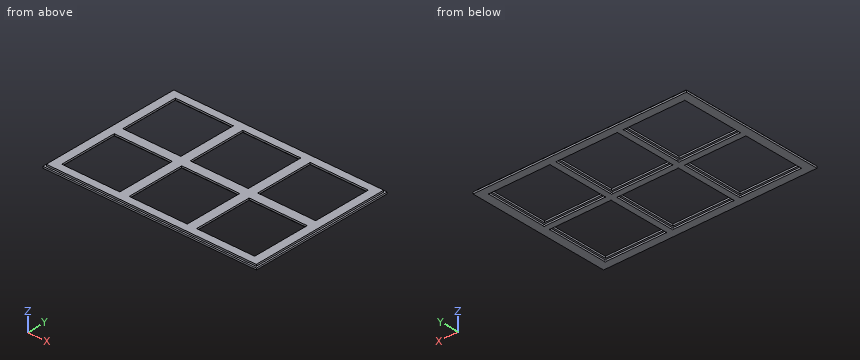
from build123d import *

# Parameters (mm, degrees)
SKETCH1_W           = 1250
SKETCH1_H           = 845
BOSS_EXTRUDE1_DEPTH = 20
SKETCH2_W           = 360
SKETCH2_H           = 360
CUT_EXTRUDE1_DEPTH  = 10
SKETCH3_W           = 340
SKETCH3_H           = 340
CUT_EXTRUDE2_DEPTH  = 11
SKETCH4_W           = 1250
SKETCH4_H           = 845
SKETCH4_W_2         = 1230
SKETCH4_H_2         = 825
CUT_EXTRUDE3_DEPTH  = 10


with BuildPart() as part:
    # Sketch1 → Boss-Extrude1 (new body)
    with BuildSketch(Plane.XY):
        Rectangle(SKETCH1_W, SKETCH1_H)
    extrude(amount=BOSS_EXTRUDE1_DEPTH)

    # Sketch2 → Cut-Extrude1 (cut)
    with BuildSketch(Plane(origin=(0, 0, 0), x_dir=(-1, 0, 0), z_dir=(0, 0, -1))):
        with Locations((-395, 197.5)):
            Rectangle(SKETCH2_W, SKETCH2_H)
        with BuildLine():
            Line((-575, 372.627718677), (-575, 377.5))
            Line((-575, 377.5), (-570.127718677, 377.5))
            ThreePointArc((-570.127718677, 377.5), (-575.474873734, 377.974873734), (-575, 372.627718677))
        make_face()
        with BuildLine():
            ThreePointArc((-215, 372.627718677), (-214.525126266, 377.974873734), (-219.872281323, 377.5))
            Line((-219.872281323, 377.5), (-215, 377.5))
            Line((-215, 377.5), (-215, 372.627718677))
        make_face()
        with BuildLine():
            Line((-180, 372.627718677), (-180, 377.5))
            Line((-180, 377.5), (-175.127718677, 377.5))
            ThreePointArc((-175.127718677, 377.5), (-180.474873734, 377.974873734), (-180, 372.627718677))
        make_face()
        with BuildLine():
            Line((-575, 17.5), (-575, 22.372281323))
            ThreePointArc((-575, 22.372281323), (-575.474873734, 17.025126266), (-570.127718677, 17.5))
            Line((-570.127718677, 17.5), (-575, 17.5))
        make_face()
        with BuildLine():
            ThreePointArc((-219.872281323, 17.5), (-214.525126266, 17.025126266), (-215, 22.372281323))
            Line((-215, 22.372281323), (-215, 17.5))
            Line((-215, 17.5), (-219.872281323, 17.5))
        make_face()
        with BuildLine():
            Line((-180, 17.5), (-180, 22.372281323))
            ThreePointArc((-180, 22.372281323), (-180.474873734, 17.025126266), (-175.127718677, 17.5))
            Line((-175.127718677, 17.5), (-180, 17.5))
        make_face()
        with Locations((0, 197.5)):
            Rectangle(SKETCH2_W, SKETCH2_H)
        with BuildLine():
            Line((180, 17.5), (175.127718677, 17.5))
            ThreePointArc((175.127718677, 17.5), (180.474873734, 17.025126266), (180, 22.372281323))
            Line((180, 22.372281323), (180, 17.5))
        make_face()
        with BuildLine():
            Line((175.127718677, -17.5), (180, -17.5))
            Line((180, -17.5), (180, -22.372281323))
            ThreePointArc((180, -22.372281323), (180.474873734, -17.025126266), (175.127718677, -17.5))
        make_face()
        with BuildLine():
            Line((215, -17.5), (219.872281323, -17.5))
            ThreePointArc((219.872281323, -17.5), (214.525126266, -17.025126266), (215, -22.372281323))
            Line((215, -22.372281323), (215, -17.5))
        make_face()
        with BuildLine():
            Line((215, 17.5), (215, 22.372281323))
            ThreePointArc((215, 22.372281323), (214.525126266, 17.025126266), (219.872281323, 17.5))
            Line((219.872281323, 17.5), (215, 17.5))
        make_face()
        with Locations((395, 197.5)):
            Rectangle(SKETCH2_W, SKETCH2_H)
        with BuildLine():
            ThreePointArc((180, 372.627718677), (180.474873734, 377.974873734), (175.127718677, 377.5))
            Line((175.127718677, 377.5), (180, 377.5))
            Line((180, 377.5), (180, 372.627718677))
        make_face()
        with BuildLine():
            Line((215, 372.627718677), (215, 377.5))
            Line((215, 377.5), (219.872281323, 377.5))
            ThreePointArc((219.872281323, 377.5), (214.525126266, 377.974873734), (215, 372.627718677))
        make_face()
        with BuildLine():
            ThreePointArc((575, 372.627718677), (575.474873734, 377.974873734), (570.127718677, 377.5))
            Line((570.127718677, 377.5), (575, 377.5))
            Line((575, 377.5), (575, 372.627718677))
        make_face()
        with BuildLine():
            Line((575, 17.5), (570.127718677, 17.5))
            ThreePointArc((570.127718677, 17.5), (575.474873734, 17.025126266), (575, 22.372281323))
            Line((575, 22.372281323), (575, 17.5))
        make_face()
        with BuildLine():
            Line((570.127718677, -17.5), (575, -17.5))
            Line((575, -17.5), (575, -22.372281323))
            ThreePointArc((575, -22.372281323), (575.474873734, -17.025126266), (570.127718677, -17.5))
        make_face()
        with Locations((395, -197.5)):
            Rectangle(SKETCH2_W, SKETCH2_H)
        with BuildLine():
            ThreePointArc((570.127718677, -377.5), (575.474873734, -377.974873734), (575, -372.627718677))
            Line((575, -372.627718677), (575, -377.5))
            Line((575, -377.5), (570.127718677, -377.5))
        make_face()
        with BuildLine():
            Line((215, -377.5), (215, -372.627718677))
            ThreePointArc((215, -372.627718677), (214.525126266, -377.974873734), (219.872281323, -377.5))
            Line((219.872281323, -377.5), (215, -377.5))
        make_face()
        with BuildLine():
            ThreePointArc((175.127718677, -377.5), (180.474873734, -377.974873734), (180, -372.627718677))
            Line((180, -372.627718677), (180, -377.5))
            Line((180, -377.5), (175.127718677, -377.5))
        make_face()
        with Locations((0, -197.5)):
            Rectangle(SKETCH2_W, SKETCH2_H)
        with BuildLine():
            Line((-180, -17.5), (-175.127718677, -17.5))
            ThreePointArc((-175.127718677, -17.5), (-180.474873734, -17.025126266), (-180, -22.372281323))
            Line((-180, -22.372281323), (-180, -17.5))
        make_face()
        with BuildLine():
            Line((-215, -17.5), (-215, -22.372281323))
            ThreePointArc((-215, -22.372281323), (-214.525126266, -17.025126266), (-219.872281323, -17.5))
            Line((-219.872281323, -17.5), (-215, -17.5))
        make_face()
        with Locations((-395, -197.5)):
            Rectangle(SKETCH2_W, SKETCH2_H)
        with BuildLine():
            ThreePointArc((-570.127718677, -17.5), (-575.474873734, -17.025126266), (-575, -22.372281323))
            Line((-575, -22.372281323), (-575, -17.5))
            Line((-575, -17.5), (-570.127718677, -17.5))
        make_face()
        with BuildLine():
            ThreePointArc((-575, -372.627718677), (-575.474873734, -377.974873734), (-570.127718677, -377.5))
            Line((-570.127718677, -377.5), (-575, -377.5))
            Line((-575, -377.5), (-575, -372.627718677))
        make_face()
        with BuildLine():
            Line((-215, -372.627718677), (-215, -377.5))
            Line((-215, -377.5), (-219.872281323, -377.5))
            ThreePointArc((-219.872281323, -377.5), (-214.525126266, -377.974873734), (-215, -372.627718677))
        make_face()
        with BuildLine():
            ThreePointArc((-180, -372.627718677), (-180.474873734, -377.974873734), (-175.127718677, -377.5))
            Line((-175.127718677, -377.5), (-180, -377.5))
            Line((-180, -377.5), (-180, -372.627718677))
        make_face()
    extrude(amount=-CUT_EXTRUDE1_DEPTH, mode=Mode.SUBTRACT)

    # Sketch3 → Cut-Extrude2 (cut, through all)
    with BuildSketch(Plane(origin=(0, 0, 10), x_dir=(-1, 0, 0), z_dir=(0, 0, -1))):
        with Locations((0, 197.5)):
            Rectangle(SKETCH3_W, SKETCH3_H)
        with Locations((395, 197.5)):
            Rectangle(SKETCH3_W, SKETCH3_H)
        with Locations((-395, 197.5)):
            Rectangle(SKETCH3_W, SKETCH3_H)
        with Locations((-395, -197.5)):
            Rectangle(SKETCH3_W, SKETCH3_H)
        with Locations((0, -197.5)):
            Rectangle(SKETCH3_W, SKETCH3_H)
        with Locations((395, -197.5)):
            Rectangle(SKETCH3_W, SKETCH3_H)
    extrude(amount=-CUT_EXTRUDE2_DEPTH, mode=Mode.SUBTRACT)

    # Sketch4 → Cut-Extrude3 (cut)
    with BuildSketch(Plane.XY.offset(20)):
        Rectangle(SKETCH4_W, SKETCH4_H)
        Rectangle(SKETCH4_W_2, SKETCH4_H_2, mode=Mode.SUBTRACT)
    extrude(amount=-CUT_EXTRUDE3_DEPTH, mode=Mode.SUBTRACT)


solid = part.part
Build history of the part. All positions in model axes, mm. Round coordinates to 2 decimals unless told otherwise and drop trailing zeros. Write each loop counter-clockwise with the first axis right and the second up, starting at its lowest first coordinate (ties: lowest second). Pieces come first, ordered by that corner, then holes. Notation, with made-up numbers: (36, -13.5) - (89, -13.5) arc R22 cw to (89, 19.5) - close; hole circle Ø3 at (88.5, 3.5). An arc over 180 degrees is marked (long way). Use CSV: the item, a comma, the result in double quotes.
(1) Wall check: line 1 (Y direction, x = -467.5, z = 18); line 2 (Y direction, x = 277, z = 9.5); line 3 (X direction, y = -323.5, z = 12.25). Give the ranges that are in metal, low to high.
Response:
line 1,"-412.5 to -367.5, -27.5 to 27.5, 367.5 to 412.5"
line 2,"-422.5 to -377.5, -17.5 to 17.5, 377.5 to 422.5"
line 3,"-615 to -565, -225 to -170, 170 to 225, 565 to 615"
(2) Band-saw the part on C-C (z = 14.25). Write the cut outline in (x, y).
Response:
outline,"(-615, -412.5) - (615, -412.5) - (615, 412.5) - (-615, 412.5) - close; hole (-565, -367.5) - (-225, -367.5) - (-225, -27.5) - (-565, -27.5) - close; hole (-565, 27.5) - (-225, 27.5) - (-225, 367.5) - (-565, 367.5) - close; hole (-170, -367.5) - (170, -367.5) - (170, -27.5) - (-170, -27.5) - close; hole (-170, 27.5) - (170, 27.5) - (170, 367.5) - (-170, 367.5) - close; hole (225, -367.5) - (565, -367.5) - (565, -27.5) - (225, -27.5) - close; hole (225, 27.5) - (565, 27.5) - (565, 367.5) - (225, 367.5) - close"
(3) Band-saw the part on A-A (y = -156.5). Give the number of separate pieces and of enclosed holes in the cut face, plus the area to 3 significant figures.
Response:
separate pieces,"4"
enclosed holes,"0"
area,"3,800 mm²"
(4) Pin check, flat tips, straight feed: P1, Ø8, axis at y = -164.5, z = 15.5, coming from the -X side; P2, Ø4, axis at x = 165.5, z = 13, coming from the +Y side; P3, Ø8, axis at y = 267, z = 16.5, coming from the +X side. Stop position of each tip, or through.
Response:
P1,"x = -615"
P2,"y = 412.5"
P3,"x = 615"
(5) Band-saw the part on B-B (x = 444.5). Write the cut outline in (y, z), plus the area to 3 significant figures.
Response:
outline,"(-422.5, 0) - (-377.5, 0) - (-377.5, 10) - (-367.5, 10) - (-367.5, 20) - (-412.5, 20) - (-412.5, 10) - (-422.5, 10) - close; (-27.5, 10) - (-17.5, 10) - (-17.5, 0) - (17.5, 0) - (17.5, 10) - (27.5, 10) - (27.5, 20) - (-27.5, 20) - close; (367.5, 10) - (377.5, 10) - (377.5, 0) - (422.5, 0) - (422.5, 10) - (412.5, 10) - (412.5, 20) - (367.5, 20) - close"
area,"2,700 mm²"
